Source: CAD feature listing. Evaluate the final solid. Frame: model axes, mm. Round coordinates to 2 decimals unless told otherwise and drop trailing zeros. Loops run counter-clockwise (first coordinate to the right, second up) from the corner with the lowest first, then second, coordinate; pieces in that order, holes last. Notation, with made-up numbers: (-29, 66) -> (3, 66) arc R19 cw to (3, 76) -> close; hole circle Ø4 at (14.25, 8). An arc over 180 degrees is marked (long way). Return JSON: item names as keys, results as strings. Group by question number.
```python
from build123d import *

# Parameters (mm, degrees)
SKETCH_1_W          = 119
SKETCH_1_H          = 63.1
EXTRUDE_1_DEPTH     = 13
SKETCH_2_R          = 1.6
CUT_EXTRUDE_2_DEPTH = 13
SKETCH_3_R          = 1
EXTRUDE_2_DEPTH     = 5.3
SKETCH_4_R          = 0.5
EXTRUDE_3_DEPTH     = 5.3


with BuildPart() as part:
    # 草图1 → 凸台-拉伸1 (new body)
    with BuildSketch(Plane(origin=(0, 0, 0), x_dir=(1, 0, 0), z_dir=(0, 1, 0))):
        Rectangle(SKETCH_1_W, SKETCH_1_H)
    extrude(amount=EXTRUDE_1_DEPTH)

    # 草图2 → 切除-拉伸2 (cut)
    with BuildSketch(Plane(origin=(0, 13, 0), x_dir=(1, 0, 0), z_dir=(0, 1, 0))):
        with Locations((53.35, 25.4)):
            Circle(SKETCH_2_R)
        with Locations((53.35, -25.4)):
            Circle(SKETCH_2_R)
        with Locations((-53.35, 25.4)):
            Circle(SKETCH_2_R)
        with Locations((-53.35, -25.4)):
            Circle(SKETCH_2_R)
    extrude(amount=-CUT_EXTRUDE_2_DEPTH, mode=Mode.SUBTRACT)

    # 草图3 → 凸台-拉伸2 (add)
    with BuildSketch(Plane(origin=(0, 13, 0), x_dir=(1, 0, 0), z_dir=(0, 1, 0))):
        with Locations((53.35, 17.78)):
            Circle(SKETCH_3_R)
        with Locations((53.35, -17.78)):
            Circle(SKETCH_3_R)
        with Locations((-53.35, 12.7)):
            Circle(SKETCH_3_R)
        with Locations((-53.35, 2.54)):
            Circle(SKETCH_3_R)
    extrude(amount=EXTRUDE_2_DEPTH)

    # 草图4 → 凸台-拉伸3 (add)
    with BuildSketch(Plane(origin=(0, 13, 0), x_dir=(1, 0, 0), z_dir=(0, 1, 0))):
        with Locations((-53.35, -7.62)):
            Circle(SKETCH_4_R)
        with Locations((-53.35, -11.43)):
            Circle(SKETCH_4_R)
        with Locations((34.3, 26.67)):
            Circle(SKETCH_4_R)
        with Locations((38.11, 26.67)):
            Circle(SKETCH_4_R)
        with Locations((30.49, 26.67)):
            Circle(SKETCH_4_R)
        with Locations((26.68, 26.67)):
            Circle(SKETCH_4_R)
        with Locations((22.87, 26.67)):
            Circle(SKETCH_4_R)
    extrude(amount=EXTRUDE_3_DEPTH)


solid = part.part
```
(1) Pin query (flat end, axial travel): pin 1 (2.5 mm diameter, centred on x = -53.35, z = 25.4, fed in from +Y); pin 2 (12 mm diameter, centred on x = 20, z = 18.5, fed in from +Y). Return the tip coordinate at first contact, or that it passes through.
(2) Cut plane A-A (y = 15). Count the separate pieces of the cut face and the enclosed holes in it, and give its area (3 significant figures).
(3) Cut plane C-C (x = -29). Return loops of the section in (y, z), and give its area (3 significant figures).
(4) Mould query, pull axis Z, two halves, no side actions, for faces 1 (the face through (-51.824, 6.591, 24.919)), 2 (the face through (-1, 6, 31.55)), 3 (the face through (-1, 0, 0)), 4 (the face through (-1, 6, -31.55)). Classes: released by +Z, released by -Z, zero draft, split by the parting line, or undercut.
(5) Ray query, line 1 (X direction, y = 8.5, z = 25.4); line 2 (Z direction, x = -53.35, y = 6.75); line 3 (Y direction, x = -9.5, z = 19). Return the intervals inside material, ascending.
(6) Cut plane B-B (z = 5). Return loops of the section in (x, y).
Answers follow:
{
 "1": {"pin 1": "through", "pin 2": "y = 13"},
 "2": {"separate pieces": "11", "enclosed holes": "0", "area": "18.1 mm^2"},
 "3": {"outline": "(0, -31.55) -> (13, -31.55) -> (13, 31.55) -> (0, 31.55) -> close", "area": "820 mm^2"},
 "4": {"face 1": "undercut", "face 2": "released by +Z", "face 3": "zero draft", "face 4": "released by -Z"},
 "5": {"line 1": "-59.5 to -54.95, -51.75 to 51.75, 54.95 to 59.5", "line 2": "-31.55 to -27, -23.8 to 23.8, 27 to 31.55", "line 3": "0 to 13"},
 "6": {"outline": "(-59.5, 0) -> (59.5, 0) -> (59.5, 13) -> (-59.5, 13) -> close"}
}
